Autodesk Inventor part; units mm, degrees
ref_plane "screw_XY" through (0, 0, 0) normal (1, 0, 0) x (0, 0, -1)
ref_plane "screw_YZ" through (0, 0, 0) normal (0, 0, -1) x (0, 1, 0)
ref_plane "screw_ZX" through (0, 0, 0) normal (0, 1, 0) x (1, 0, 0)
sketch "Sketch_1" plane through (0, 0, 0) normal (0, 0, 1) x (1, 0, 0)
  line L0 (9.525, 0) -> (-3.2258, 0)
  line L1 (-3.2258, 0) -> (-3.2258, 4.6101)
  line L2 (-3.2258, 4.6101) -> (-3.0734, 4.7625)
  line L3 (-3.0734, 4.7625) -> (-0.254, 4.7625)
  arc A0 (0, 4.5085) -> (-0.254, 4.7625) centre (-0.254, 4.5085) ccw
  line L4 (0, 4.5085) -> (0, 3.2512)
  arc A1 (0, 3.2512) -> (0.0762, 3.175) centre (0.0762, 3.2512) ccw
  line L5 (0.0762, 3.175) -> (8.7693, 3.175)
  line L6 (8.7693, 3.175) -> (9.525, 2.4194)
  line L7 (9.525, 2.4194) -> (9.525, 0)
  line L8 (9.525, 0) -> (-3.2258, 0)
revolve "Revolution1" add sketch "Sketch_1" angle 360 about axis through (9.525, 0, 0) along (1, 0, 0)
thread "Thread1"
sketch "Sketch_3" plane through (-3.2258, 0, 0) normal (1, 0, 0) x (0, 0, -1)
  line L0 (-1.5875, -0.9165) -> (0, -1.8331)
  line L1 (0, -1.8331) -> (1.5875, -0.9165)
  line L2 (1.5875, -0.9165) -> (1.5875, 0.9165)
  line L3 (1.5875, 0.9165) -> (0, 1.8331)
  line L4 (0, 1.8331) -> (-1.5875, 0.9165)
  line L5 (-1.5875, 0.9165) -> (-1.5875, -0.9165)
extrude "Extrusion1" cut sketch "Sketch_3" along normal blind 1.6256
sketch "Sketch_4" plane through (0, 0, 0) normal (0, 0, 1) x (1, 0, 0)
  line L0 (-0.6837, 0) -> (-1.6002, 0)
  line L1 (-1.6002, 0) -> (-1.6002, 1.5875)
  line L2 (-1.6002, 1.5875) -> (-0.6837, 0)
  line L3 (-0.6837, 0) -> (-1.6002, 0)
revolve "Revolution2" cut sketch "Sketch_4" angle 360 about axis through (-0.6837, 0, 0) along (1, 0, 0)
ref_plane "screw_XY" through (0, 0, 0) normal (1, 0, 0) x (0, 0, -1)
ref_plane "screw_YZ" through (0, 0, 0) normal (0, 0, -1) x (0, 1, 0)
ref_plane "screw_ZX" through (0, 0, 0) normal (0, 1, 0) x (1, 0, 0)
ref_plane "screw1_XY" through (9.525, 0, 0) normal (1, 0, 0) x (0, 0, -1)
ref_plane "screw1_YZ" through (9.525, 0, 0) normal (0, 0, -1) x (0, 1, 0)
ref_plane "screw1_ZX" through (9.525, 0, 0) normal (0, 1, 0) x (1, 0, 0)
ref_plane "screw2_XY" through (4.445, 0, 0) normal (1, 0, 0) x (0, 0, -1)
ref_plane "screw2_YZ" through (4.445, 0, 0) normal (0, 0, -1) x (0, 1, 0)
ref_plane "screw2_ZX" through (4.445, 0, 0) normal (0, 1, 0) x (1, 0, 0)
ref_plane "to_tnut_XY" through (7.366, 0, 0) normal (1, 0, 0) x (0, 0, -1)
ref_plane "to_tnut_YZ" through (7.366, 0, 0) normal (0, 0, -1) x (0, 1, 0)
ref_plane "to_tnut_ZX" through (7.366, 0, 0) normal (0, 1, 0) x (1, 0, 0)
properties part number "2750-0.250"
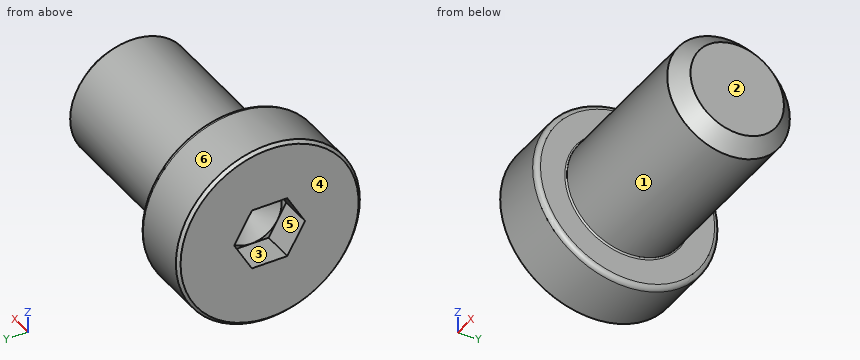
Can you work these out from the model? Positions are in its coordinate system, mm. Face numbers are marked on the shaded views. A direction names the side the tool comes from. Coordinates: 2 decimals unless noted, no trailing zeros. Loops run counter-clockwise (first coordinate to the right, second up) from the corner with the lowest first, then second, coordinate; pieces in that order, holes last. Notation, with made-up numbers: (7.25, 66) -> (66.25, 66) arc R29 ccw to (66.25, 90) -> close; hole circle Ø4 at (30.5, 10.5). An arc over 180 degrees is marked (long way). Answer as a JSON object with one key per item and string values.
1) Imagine slicing it at A-A (x = 5.5). Please give me the cut outline in (y, z) (3 decimals), then the cut area to 3 significant figures.
Results:
{"outline": "circle Ø6.35 at (0, 0)", "area": "31.7 mm^2"}
2) For P1, Ø1.5, axis at y = -3.5, z = 2.5, coming from the +X side; P2, Ø1.8, axis at x = -2.5, y = 0.5, coming from the +Z side; P3, Ø1, axis at x = 4.5, y = 2.5, coming from the -Z side; P4, Ø3, axis at x = 5.5, z = 3.5, coming from the -Y side, each with a flat end and sliding along its axis, tell me the tip position at first contact or that it passes through.
Results:
{"P1": "stops at x = 0", "P2": "stops at z = 4.76", "P3": "stops at z = -2.47", "P4": "stops at y = -2.47"}
3) For the marked faces 1, 2 and 3, which set-ups out of +Z, -Z, +X, -X, +Y, -Y let a thin tool reach every point of the face, with its end or its side?
Results:
{"face 1": "+X", "face 2": "+Z, -Z, +X, +Y, -Y", "face 3": "-X"}
4) If I drill on line 1 (X direction, y = 3.25, z = -2); line 2 (Y direction, x = 1.5, z = 2.75); line 3 (Y direction, x = -2.5, z = 1.5), over which ranges is the centre line in solid material (lowest first)?
Results:
{"line 1": "x = -3.23 to 0", "line 2": "y = -1.59 to 1.59", "line 3": "y = -4.52 to -0.97, 0.97 to 4.52"}
5) Thinking about a two-plate mould opening in Y: for the marked faces 4, 5 and 6, which applies, pulls with the +Y half, pulls with the -Y half, needs draft (parallel to the pull), parting line crosses it, or undercut?
Results:
{"face 4": "needs draft", "face 5": "undercut", "face 6": "parting line crosses it"}
